Geometry: final body of the model. Coordinates: model frame, mm. Face numbers are marked on the shaded views. A direction names the side the tool comes from. Round coordinates to 2 decimals unless told otherwise and drop trailing zeros. Loops run counter-clockwise (first coordinate to the right, second up) from the corner with the lowest first, then second, coordinate; pieces in that order, holes last. Notation, with made-up numbers: (36.25, 2.5) - (43.25, 2.5) arc R14 ccw to (43.25, 7.5) - close; hole circle Ø3 at (63, 9). An arc over 180 degrees is marked (long way). Return JSON: item names as keys, results as strings. Group by question number.
1. Material intervals for probe 1 along Z at (x, y) = (8.3, -3.6); probe 2 along Z at (x, y) = (7.25, -4.5); probe 3 along X at (y, z) = (-3.3, 13.6), sorted ascending.
2. Section C-C on x = 0.5. Return loops of the section in (y, z).
3. First-contact query: pin 1 Ø0.8 at (x, y) = (7, -1.5) entering from +Z; pin 2 Ø1.5 at (y, z) = (-2.5, 7) entering from +X; pin 3 Ø1 at (x, z) = (9.5, 2.5) entering from -Y. Flat tips, straight axial feed; report the tip coordinate or a pass-through.
4. Section A-A on y = 1. Return loops of the section in (x, z).
5. Draft query along Z for the marked faces 3, 4, 5 and 6. Return one class per face: +Z half, -Z half, draft (parallel to the pull), parting line (faces both ways), or undercut.
6. Set-up query: the marked faces 1 and 2. Return all of +Z, -Z, +X, -X, +Y, -Y with unobstructed straight access to the full face (end or side cutting, diameter ignored); none if empty.
7. Section D-D on y = -3.5. Return loops of the section in (x, z).
8. Section B-B on z = 7.5. Return loops of the section in (x, y).
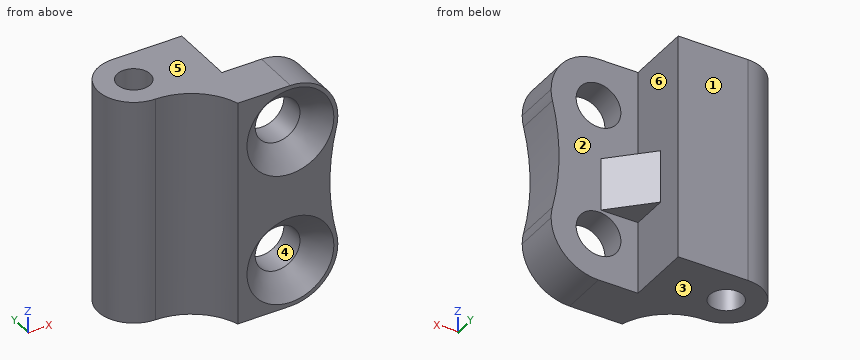
from build123d import *

# Parameters (mm, degrees)
SKETCH_1_R                = 1.25
EXTRUDE_1_DEPTH           = 17.2
CUT_EXTRUDE_1_DEPTH       = 9.6
EXTRUDE_2_DEPTH           = 4
HOLE_WIZARD_1_D           = 3.4
HOLE_WIZARD_1_DEPTH       = 8.6
HOLE_WIZARD_1_CSINK_D     = 6.6
HOLE_WIZARD_1_CSINK_ANGLE = 90
HOLE_WIZARD_1_TIP         = 1.021463052


with BuildPart() as part:
    # 草图1 → 凸台-拉伸1 (new body)
    with BuildSketch(Plane.XY):
        with BuildLine():
            Line((0, 2.7), (5.3, 2.7))
            Line((5.3, 2.7), (5.3, -2.3))
            Line((5.3, -2.3), (12.8, -2.3))
            Line((12.8, -2.3), (12.8, -5.9))
            Line((12.8, -5.9), (4.3, -5.9))
            ThreePointArc((4.3, -5.9), (2.680018657, -3.58778743), (0, -2.7))
            ThreePointArc((0, -2.7), (-2.7, 0), (0, 2.7))
        make_face()
        Circle(SKETCH_1_R, mode=Mode.SUBTRACT)
    extrude(amount=EXTRUDE_1_DEPTH)

    # 草图6 → 切除-拉伸1 (cut, through all)
    with BuildSketch(Plane.XZ.offset(5.9)):
        with BuildLine():
            Line((8.3, 0), (12.8, 0))
            Line((12.8, 0), (12.8, 17.2))
            Line((12.8, 17.2), (8.3, 17.2))
            ThreePointArc((8.3, 17.2), (10.845584412, 16.145584412), (11.9, 13.6))
            ThreePointArc((11.9, 13.6), (11.874356619, 13.171077206), (11.797791798, 12.748264984))
            ThreePointArc((11.797791798, 12.748264984), (11.3, 8.6), (11.797791798, 4.451735016))
            ThreePointArc((11.797791798, 4.451735016), (11.874356619, 4.028922794), (11.9, 3.6))
            ThreePointArc((11.9, 3.6), (10.845584412, 1.054415588), (8.3, 0))
        make_face()
    extrude(amount=-CUT_EXTRUDE_1_DEPTH, mode=Mode.SUBTRACT)

    # 草图7 → 凸台-拉伸2 (add)
    with BuildSketch(Plane.XY.offset(5.5)):
        Polygon((8.128427125, -2.3), (5.3, -2.3), (5.3, 0.528427125), align=None)
    extrude(amount=EXTRUDE_2_DEPTH)

    # 打孔尺寸(%根据)开槽半沉头木螺钉的类型1
    with Locations(Plane(origin=(8.3, -5.9, 3.6), x_dir=(-1, 0, 0), z_dir=(0, -1, 0))):
        with Locations((0, 0), (0, -10)):
            CounterSinkHole(HOLE_WIZARD_1_D / 2, HOLE_WIZARD_1_CSINK_D / 2, depth=HOLE_WIZARD_1_DEPTH, counter_sink_angle=HOLE_WIZARD_1_CSINK_ANGLE)
            with Locations((0, 0, -(HOLE_WIZARD_1_DEPTH + HOLE_WIZARD_1_TIP / 2))):  # 118° drill point
                Cone(0, HOLE_WIZARD_1_D / 2, HOLE_WIZARD_1_TIP, mode=Mode.SUBTRACT)


solid = part.part
Taken from the geometry:
{
 "1": {"probe 1": "0 to 1.9, 5.3 to 11.9, 15.3 to 17.2", "probe 2": "0 to 2.02, 5.18 to 12.02, 15.18 to 17.2", "probe 3": "2.24 to 6.6, 10 to 11.9"},
 "2": {"outline": "(-2.73, 0) - (-1.15, 0) - (-1.15, 17.2) - (-2.73, 17.2) - close; (1.15, 0) - (2.7, 0) - (2.7, 17.2) - (1.15, 17.2) - close"},
 "3": {"pin 1": "z = 9.5", "pin 2": "x = 11.46", "pin 3": "y = -4.73"},
 "4": {"outline": "(-2.51, 0) - (-0.75, 0) - (-0.75, 17.2) - (-2.51, 17.2) - close; (0.75, 0) - (5.3, 0) - (5.3, 17.2) - (0.75, 17.2) - close"},
 "5": {"face 3": "-Z half", "face 4": "undercut", "face 5": "+Z half", "face 6": "draft"},
 "6": {"face 1": "+Z, -Z, +X, -X, +Y", "face 2": "+X, +Y"},
 "7": {"outline": "(2.56, 0) - (8.3, 0) arc R3.6 ccw to (11.8, 4.45) arc R17.53 cw to (11.8, 12.75) arc R3.6 ccw to (8.3, 17.2) - (2.56, 17.2) - close; hole circle Ø3.4 at (8.3, 3.6); hole circle Ø3.4 at (8.3, 13.6)"},
 "8": {"outline": "(0, -2.7) arc R4.49 cw to (4.3, -5.9) - (11.33, -5.9) - (11.33, -2.3) - (8.13, -2.3) - (5.3, 0.53) - (5.3, 2.7) - (0, 2.7) arc R2.7 ccw to start; hole circle Ø2.5 at (0, 0)"}
}
